Build history of the part. All positions in model axes, mm. Face numbers are marked on the shaded views. Give positions to 0.01 mm unless a question says otherwise; leave off trailing zeros. Order: outer loops, then holes, each group sorted by start corner. A loop starts at its lowest first (then second) coordinate and runs counter-clockwise, first axis right, second up. Notation, with made-up numbers: (77.5, 59) - (136.5, 59) arc R14 cw to (136.5, 75) - close; hole circle Ø8 at (31.5, 16.25). An arc over 180 degrees is marked (long way). One line per item, written item: value.
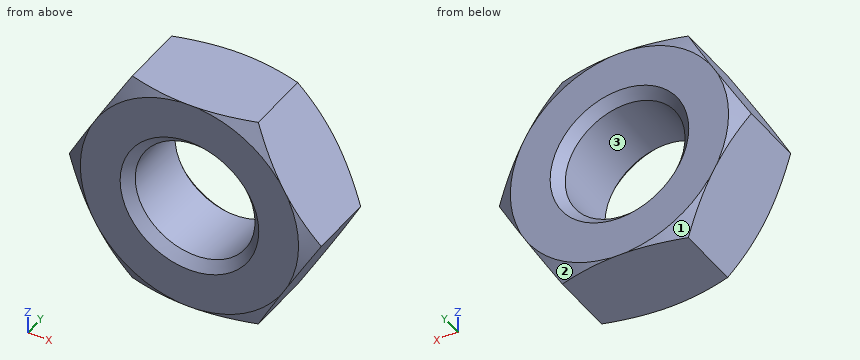
```python
from build123d import *

# Parameters (mm, degrees)
BOSS_EXTRUDE1_DEPTH     = 2.475
SKETCH2_OUTSIDE_W       = 37.888
SKETCH2_OUTSIDE_H       = 35.916
SKETCH2_OUTSIDE_R       = 6.375
CUT_EXTRUDE1_DEPTH      = 4.95
CUT_EXTRUDE1_DRAFT      = -60
MIRROR1_COPY_1_SKETCH_W = 37.888
MIRROR1_COPY_1_SKETCH_H = 35.916
MIRROR1_COPY_1_SKETCH_R = 6.375
MIRROR1_COPY_1_DEPTH    = 4.95
MIRROR1_COPY_1_DRAFT    = -60


with BuildPart() as part:
    # Sketch1 → Boss-Extrude1 (new, symmetric)
    with BuildSketch(Plane(origin=(0, 0, 0), x_dir=(1, 0, 0), z_dir=(0, 1, 0))):
        Polygon((3.680607966, -6.375), (7.361215932, 0), (3.680607966, 6.375), (-3.680607966, 6.375), (-7.361215932, 0), (-3.680607966, -6.375), align=None)
    extrude(amount=BOSS_EXTRUDE1_DEPTH, both=True)


with BuildPart() as cut_extrude1_tool:
    # Sketch2 outside → Cut-Extrude1 (with draft: the straight prism first)
    with BuildSketch(Plane(origin=(0, 2.475, 0), x_dir=(1, 0, 0), z_dir=(0, 1, 0))):
        Rectangle(SKETCH2_OUTSIDE_W, SKETCH2_OUTSIDE_H)
        Circle(SKETCH2_OUTSIDE_R, mode=Mode.SUBTRACT)
    extrude(amount=-CUT_EXTRUDE1_DEPTH)
    # Cut-Extrude1: the draft: its side faces are tilted about the plane it starts from
    cut_extrude1_sides = [cut_extrude1_tool.faces().sort_by_distance(p)[0] for p in [
        (0, 0, 17.958),
        (18.944, 0, 0),
        (0, 0, -17.958),
        (-18.944, 0, 0),
        (-6.375, 0, 0),
    ]]
    draft(cut_extrude1_sides, Plane(origin=(0, 2.475, 0), x_dir=(1, 0, 0), z_dir=(0, 1, 0)), CUT_EXTRUDE1_DRAFT)


with BuildPart() as part_1:
    add(part.part)

    # Cut-Extrude1: cut by cut_extrude1_tool
    add(cut_extrude1_tool.part, mode=Mode.SUBTRACT)


with BuildPart() as mirror1_copy_1_tool:
    # Mirror1 copy 1 sketch → Mirror1 copy 1 (with draft: the straight prism first)
    with BuildSketch(Plane.XZ.offset(2.475)):
        Rectangle(MIRROR1_COPY_1_SKETCH_W, MIRROR1_COPY_1_SKETCH_H)
        Circle(MIRROR1_COPY_1_SKETCH_R, mode=Mode.SUBTRACT)
    extrude(amount=-MIRROR1_COPY_1_DEPTH)
    # Mirror1 copy 1: the draft: its side faces are tilted about the plane it starts from
    mirror1_copy_1_sides = [mirror1_copy_1_tool.faces().sort_by_distance(p)[0] for p in [
        (0, 0, 17.958),
        (18.944, 0, 0),
        (0, 0, -17.958),
        (-18.944, 0, 0),
        (-6.375, 0, 0),
    ]]
    draft(mirror1_copy_1_sides, Plane.XZ.offset(2.475), MIRROR1_COPY_1_DRAFT)


with BuildPart() as part_2:
    add(part_1.part)

    # Mirror1 copy 1: cut by mirror1_copy_1_tool
    add(mirror1_copy_1_tool.part, mode=Mode.SUBTRACT)

    # Sketch5 → M8x1.0 Tapped Hole1 (revolve, cut)
    with BuildSketch(Plane(origin=(0, 2.475, 0), x_dir=(0, 0, 1), z_dir=(1, 0, 0))):
        Polygon((0, 0), (0, 4.95), (4.05, 4.95), (3.5, 4.4), (3.5, 0.55), (4.05, 0), align=None)
    revolve(axis=Axis((0, 8.825, 0), (0, -1, 0)), mode=Mode.SUBTRACT)


solid = part_2.part
```
(1) Drill centre lines: line 1 (Z direction, x = 0, y = 0.05) (3 decimals); line 2 (X direction, y = 0.6, z = 0.25); line 3 (X direction, y = -1.15, z = 1). Where is each one in solid material? Low to high.
Completed:
line 1: -6.375 to -3.5, 3.5 to 6.375
line 2: -7.22 to -3.49, 3.49 to 7.22
line 3: -6.78 to -3.35, 3.35 to 6.78
(2) Slice it at A-A, the plane y = 0.9. Give the cut face in (x, z) (3 decimals), and give its area (3 significant figures).
Completed:
outline: (-7.361, 0) - (-3.681, -6.375) - (3.681, -6.375) - (7.361, 0) - (3.681, 6.375) - (-3.681, 6.375) - close; hole circle Ø7 at (0, 0)
area: 102 mm²
(3) Pull direction X, two halves, no side cores. Call the marked faces 1, 2 and 3: +X half, -X half, draft (parallel to the pull), parting line (faces both ways), or undercut.
Completed:
face 1: -X half
face 2: +X half
face 3: undercut
